```python
from build123d import *

# Parameters (mm, degrees)
SKETCH2_W             = 33
SKETCH2_H             = 17
BOSS_EXTRUDE1_DEPTH   = 2
M5_TAPPED_HOLE1_D     = 4.2
F_2_0MM_DOWEL_HOLE1_D = 2
SKETCH6_R             = 8
CUT_EXTRUDE1_DEPTH    = 35.135758377


with BuildPart() as part:
    # Sketch2 → Boss-Extrude1 (new, symmetric)
    with BuildSketch(Plane(origin=(0, 0, 0), x_dir=(1, 0, 0), z_dir=(0, 1, 0))):
        Rectangle(SKETCH2_W, SKETCH2_H)
    extrude(amount=BOSS_EXTRUDE1_DEPTH, both=True)

    # M5 Tapped Hole1 (through all)
    with Locations(Plane(origin=(0.5, 2, 0), x_dir=(0, 0, 1), z_dir=(0, 1, 0))):
        with Locations((0, 0)):
            Hole(M5_TAPPED_HOLE1_D / 2)

    # Ø2.0mm Dowel Hole1 (through all)
    with Locations(Plane(origin=(-12.5, 2, 0), x_dir=(0, 0, 1), z_dir=(0, 1, 0))):
        with Locations((0, 0)):
            Hole(F_2_0MM_DOWEL_HOLE1_D / 2)

    # Sketch6 → Cut-Extrude1 (cut, through all)
    with BuildSketch(Plane(origin=(16.5, 0, 0), x_dir=(0, 0, -1), z_dir=(1, 0, 0))):
        with Locations((0, -9)):
            Circle(SKETCH6_R)
    extrude(amount=-CUT_EXTRUDE1_DEPTH, mode=Mode.SUBTRACT)


solid = part.part
```
CAD build for the part. Positions are in the model's coordinates, mm. Give positions to 0.01 mm unless a question says otherwise; leave off trailing zeros. Order: outer loops, then holes, each group sorted by start corner. A loop starts at its lowest first (then second) coordinate and runs counter-clockwise, first axis right, second up. Notation, with made-up numbers: M 40.25,-25.5 L 78.25,-25.5 A33 cw 78.25,10.5 Z; hole C 25.25,-40 d8. An arc over 180 degrees is marked long. Put each result on its own line as item: value. Start each with the question number.
(1) Saw through at A-A, the plane x = 0.5. Write the cut outline in (y, z), then the cut area to 3 significant figures.
(2) Saw through at D-D, the plane x = -12.5. Write the cut outline in (y, z).
(3) Saw through at B-B, the plane z = 0. Write the cut outline in (x, y).
(4) Saw through at C-C, the plane y = 1.4. Write the cut outline in (x, z).
(5) Flat gauge pins, fed straight in: pin 1 Ø1.5 at (x, z) = (6.5, -2) entering from -Y; pin 2 Ø4 at (x, z) = (10, -0.5) entering from -Y. Where does each tip first touch, or does it go through?
(6) Drill centre lines: line 1 along X through (y, z) = (-0.25, 0); line 2 along Z through (x, y) = (-12.5, 0.3); line 3 along X through (y, z) = (1.45, -1.25). Where is each one in solid material? Low to high.
(7) Mould opens along Z. For faces 1 (the flat face through (0, -2, -6)), 2 (the flat face through (0, 0, -8.5)), 3 (the cylindrical face through (0.23, -1.43, 2.59)) say: +Z half, -Z half, draft (parallel to the pull), parting line (faces both ways), or undercut.
Check result:
1. outline: M -2,-8.5 L 2,-8.5 L 2,-2.1 L -1.28,-2.1 A8 cw -2,-3.87 Z; M -2,3.87 A8 cw -1.28,2.1 L 2,2.1 L 2,8.5 L -2,8.5 Z
1. area: 49.8 mm2
2. outline: M -2,-8.5 L 2,-8.5 L 2,-1 L -1.06,-1 A8 cw -2,-3.87 Z; M -2,3.87 A8 cw -1.06,1 L 2,1 L 2,8.5 L -2,8.5 Z
3. outline: M -16.5,-1 L -13.5,-1 L -13.5,2 L -16.5,2 Z; M -11.5,-1 L -1.6,-1 L -1.6,2 L -11.5,2 Z; M 2.6,-1 L 16.5,-1 L 16.5,2 L 2.6,2 Z
4. outline: M -16.5,-8.5 L 16.5,-8.5 L 16.5,8.5 L -16.5,8.5 Z; hole C -12.5,0 d2; hole C 0.5,0 d4.2
5. pin 1: stops at y = -1.49
5. pin 2: stops at y = -1.4
6. line 1: x = -16.5 to -13.5, -11.5 to -1.6, 2.6 to 16.5
6. line 2: z = -8.5 to -1, 1 to 8.5
6. line 3: x = -16.5 to -1.19, 2.19 to 16.5
7. face 1: draft
7. face 2: -Z half
7. face 3: undercut
